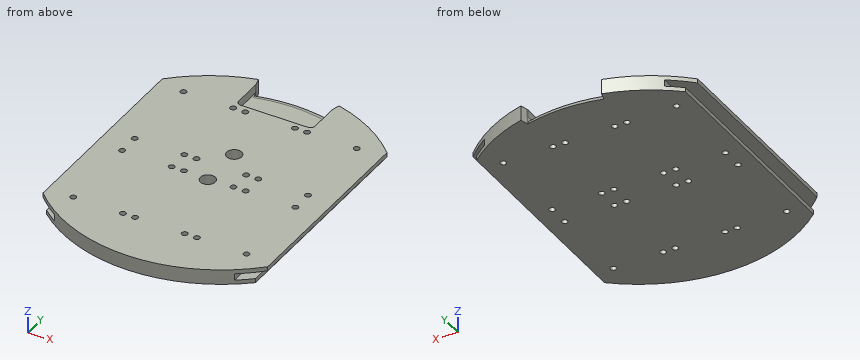
from build123d import *

# Parameters (mm, degrees)
RESSALTO_EXTRUS_O1_DEPTH = 8
ESBO_O5_R                = 4
CORTE_EXTRUS_O3_DEPTH    = 5.6
ESBO_O7_R                = 1.6
CORTE_EXTRUS_O4_DEPTH    = 180.714977127
CORTE_EXTRUS_O6_DEPTH    = 180.714977127
CORTE_EXTRUS_O7_DEPTH    = 4.4
FILETE1_R                = 2.4
FILETE2_R                = 4.4
ESBO_O11_W               = 3.5
ESBO_O11_H               = 150
CORTE_EXTRUS_O8_DEPTH    = 12
ESBO_O12_W               = 3.5
ESBO_O12_H               = 150
CORTE_EXTRUS_O9_DEPTH    = 12
ESBO_O13_W               = 4.4
ESBO_O13_H               = 156.816425971
CORTE_EXTRUS_O10_DEPTH   = 5.75


with BuildPart() as part:
    # Esboço1 → Ressalto-extrusão1 (new body)
    with BuildSketch(Plane.XY):
        with BuildLine():
            Line((0, 0), (0, -108.75))
            ThreePointArc((0, -108.75), (60, -133.542027106), (120, -108.75))
            Line((120, -108.75), (120, 0))
            ThreePointArc((120, 0), (60, 24.792027106), (0, 0))
        make_face()
    extrude(amount=RESSALTO_EXTRUS_O1_DEPTH)

    # Esboço5 → Corte-extrusão3 (cut)
    with BuildSketch(Plane.XY.offset(8)):
        with Locations((60, -60.875)):
            Circle(ESBO_O5_R)
        with Locations(Location((60, -36.875, 0), (0, 0, 180))):
            Circle(ESBO_O5_R)
    extrude(amount=-CORTE_EXTRUS_O3_DEPTH, mode=Mode.SUBTRACT)

    # Esboço7 → Corte-extrusão4 (cut, through all)
    with BuildSketch(Plane(origin=(0, 0, 0), x_dir=(-1, 0, 0), z_dir=(0, 0, -1))):
        with Locations((-73.25, -48.625)):
            Circle(ESBO_O7_R)
        with Locations((-79.75, -48.625)):
            Circle(ESBO_O7_R)
        with Locations((-106.25, -48.625)):
            Circle(ESBO_O7_R)
        with Locations(Location((-73.25, -4.125, 0), (0, 0, 180))):
            Circle(ESBO_O7_R)
        with Locations(Location((-106.25, -4.125, 0), (0, 0, 180))):
            Circle(ESBO_O7_R)
        with Locations(Location((-79.75, -4.125, 0), (0, 0, 180))):
            Circle(ESBO_O7_R)
        with Locations((-40.25, -4.125)):
            Circle(ESBO_O7_R)
        with Locations((-13.75, -4.125)):
            Circle(ESBO_O7_R)
        with Locations((-46.75, -4.125)):
            Circle(ESBO_O7_R)
        with Locations(Location((-13.75, -48.625, 0), (0, 0, 180))):
            Circle(ESBO_O7_R)
        with Locations(Location((-40.25, -48.625, 0), (0, 0, 180))):
            Circle(ESBO_O7_R)
        with Locations(Location((-46.75, -48.625, 0), (0, 0, 180))):
            Circle(ESBO_O7_R)
        with Locations((-46.75, -60.125)):
            Circle(ESBO_O7_R)
        with Locations((-40.25, -60.125)):
            Circle(ESBO_O7_R)
        with Locations((-13.75, -60.125)):
            Circle(ESBO_O7_R)
        with Locations(Location((-46.75, -104.625, 0), (0, 0, 180))):
            Circle(ESBO_O7_R)
        with Locations(Location((-13.75, -104.625, 0), (0, 0, 180))):
            Circle(ESBO_O7_R)
        with Locations(Location((-40.25, -104.625, 0), (0, 0, 180))):
            Circle(ESBO_O7_R)
        with Locations((-79.75, -104.625)):
            Circle(ESBO_O7_R)
        with Locations((-106.25, -104.625)):
            Circle(ESBO_O7_R)
        with Locations((-73.25, -104.625)):
            Circle(ESBO_O7_R)
        with Locations(Location((-106.25, -60.125, 0), (0, 0, 180))):
            Circle(ESBO_O7_R)
        with Locations(Location((-79.75, -60.125, 0), (0, 0, 180))):
            Circle(ESBO_O7_R)
        with Locations(Location((-73.25, -60.125, 0), (0, 0, 180))):
            Circle(ESBO_O7_R)
    extrude(amount=-CORTE_EXTRUS_O4_DEPTH, mode=Mode.SUBTRACT)

    # Esboço9 → Corte-extrusão6 (cut, through all)
    with BuildSketch(Plane.XY.offset(8)):
        with BuildLine():
            Line((39.6, 17.767664327), (38.486352357, 22.024398865))
            ThreePointArc((38.486352357, 22.024398865), (60, 24.792027106), (81.513647643, 22.024398865))
            Line((81.513647643, 22.024398865), (80.4, 17.767664327))
            ThreePointArc((80.4, 17.767664327), (60, 20.392027106), (39.6, 17.767664327))
        make_face()
    extrude(amount=-CORTE_EXTRUS_O6_DEPTH, mode=Mode.SUBTRACT)

    # Esboço10 → Corte-extrusão7 (cut)
    with BuildSketch(Plane.XY.offset(8)):
        with BuildLine():
            Line((39.6, 17.767664327), (39.6, -0.432335673))
            Line((39.6, -0.432335673), (80.4, -0.432335673))
            Line((80.4, -0.432335673), (80.4, 17.767664327))
            ThreePointArc((80.4, 17.767664327), (60, 20.392027106), (39.6, 17.767664327))
        make_face()
    extrude(amount=-CORTE_EXTRUS_O7_DEPTH, mode=Mode.SUBTRACT)

    # Filete1
    filete1_edges = [part.edges().sort_by_distance(p)[0] for p in [
        (80.4, -0.432335673, 5.8),
        (39.6, -0.432335673, 5.8),
        (39.6, 17.767664327, 5.8),
        (80.4, 17.767664327, 5.8),
    ]]
    fillet(filete1_edges, radius=FILETE1_R)

    # Filete2
    # the kernel refuses this fillet: 4.4 mm, written as the material it takes off along each edge
    with BuildSketch(Plane(origin=(60, -60.207972894, 3.6), x_dir=(0.25310173697270616, 0.9674396677526714, 0), z_dir=(0.9674396677526714, -0.25310173697270616, 0))) as filete2_piece_1:
        with BuildLine():
            CenterArc((76.273338469, -4.4), FILETE2_R, 10.475681696, 79.524318304)
            Line((80.6, -3.6), (80.6, 0))
            Line((80.6, 0), (76.273338469, 0))
        make_face()
    revolve(axis=Axis((60, -60.207972894, 3.6), (0, 0, 1)), revolution_arc=29.322266437, mode=Mode.SUBTRACT)

    # Esboço11 → Corte-extrusão8 (cut)
    with BuildSketch(Plane.ZY):
        with Locations((4, -53.75)):
            Rectangle(ESBO_O11_W, ESBO_O11_H)
    extrude(amount=-CORTE_EXTRUS_O8_DEPTH, mode=Mode.SUBTRACT)

    # Esboço12 → Corte-extrusão9 (cut)
    with BuildSketch(Plane(origin=(120, 0, 0), x_dir=(0, 0, -1), z_dir=(1, 0, 0))):
        with Locations((-4, -53.75)):
            Rectangle(ESBO_O12_W, ESBO_O12_H)
    extrude(amount=-CORTE_EXTRUS_O9_DEPTH, mode=Mode.SUBTRACT)

    # Esboço13 → Corte-extrusão10 (cut)
    with BuildSketch(Plane(origin=(0, 0, 0), x_dir=(-1, 0, 0), z_dir=(0, 0, -1))):
        with Locations((-118, -55.758814121)):
            Rectangle(ESBO_O13_W, ESBO_O13_H)
        with Locations((-2, -55.758814121)):
            Rectangle(ESBO_O13_W, ESBO_O13_H)
    extrude(amount=-CORTE_EXTRUS_O10_DEPTH, mode=Mode.SUBTRACT)


solid = part.part
Model file for the job. Use its own axes, mm. Give positions to 0.01 mm unless a question says otherwise; leave off trailing zeros. Order: outer loops, then holes, each group sorted by start corner. A loop starts at its lowest first (then second) coordinate and runs counter-clockwise, first axis right, second up. Notation, with made-up numbers: (43, -0.75) - (69, -0.75) arc R9 cw to (69, 5.25) - close; hole circle Ø5 at (-28, 4). An arc over 180 degrees is marked (long way). One line per item, written item: value.
Item 1: Slice it at C-C (x = 106.25). List the corners of the cut face in (y, z) (3 decimals), then the cut area to 3 significant figures.
Response values:
outline: (-119.858, 0) - (-106.225, 0) - (-106.225, 8) - (-119.858, 8) - close; (-103.025, 0) - (-61.725, 0) - (-61.725, 8) - (-103.025, 8) - close; (-58.525, 0) - (-50.225, 0) - (-50.225, 8) - (-58.525, 8) - close; (-47.025, 0) - (-5.725, 0) - (-5.725, 8) - (-47.025, 8) - close; (-2.525, 0) - (11.108, 0) - (11.108, 8) - (-2.525, 8) - close
area: 945 mm2
Item 2: Slice it at D-D (x = 60). List the corners of the cut face in (y, z) (3 decimals).
Response values:
outline: (-133.542, 0) - (20.392, 0) arc R4.4 ccw to (16.065, 3.6) - (-0.432, 3.6) - (-0.432, 8) - (-32.875, 8) - (-32.875, 2.4) - (-40.875, 2.4) - (-40.875, 8) - (-56.875, 8) - (-56.875, 2.4) - (-64.875, 2.4) - (-64.875, 8) - (-133.542, 8) - close
Item 3: Slice it at A-A (x = 10). List the corners of the cut face in (y, z).
Response values:
outline: (-117.28, 0) - (8.53, 0) - (8.53, 2.25) - (-117.28, 2.25) - close; (-117.28, 5.75) - (8.53, 5.75) - (8.53, 8) - (-117.28, 8) - close
Item 4: Slice it at B-B (y = -21.5). List the corners of the cut face in (x, z).
Response values:
outline: (0, 5.75) - (12, 5.75) - (12, 2.25) - (4.2, 2.25) - (4.2, 0) - (115.8, 0) - (115.8, 2.25) - (108, 2.25) - (108, 5.75) - (120, 5.75) - (120, 8) - (0, 8) - close
Item 5: Pin check, flat tips, straight feed: pin 1 Ø5.5 at (x, y) = (51.5, 7) entering from +Z; pin 2 Ø1.9 at (x, y) = (79.75, -48.625) entering from +Z; pin 3 Ø1 at (y, z) = (-63, 5) entering from -X; pin 4 Ø4 at (x, z) = (81.5, 7) entering from -Y. Stop position of each tip, or through.
Response values:
pin 1: z = 3.6
pin 2: through
pin 3: x = 12
pin 4: y = -131.28
Item 6: Wall check: line 1 (Y direction, x = 61, z = 2.5); line 2 (Z direction, x = 109.5, y = -53); line 3 (X direction, y = -68, z = 3.5). Give the ranges that are in metal, low to high.
Response values:
line 1: -133.54 to -64.75, -57 to -40.75, -33 to 18.97
line 2: 0 to 2.25, 5.75 to 8
line 3: 12 to 108
